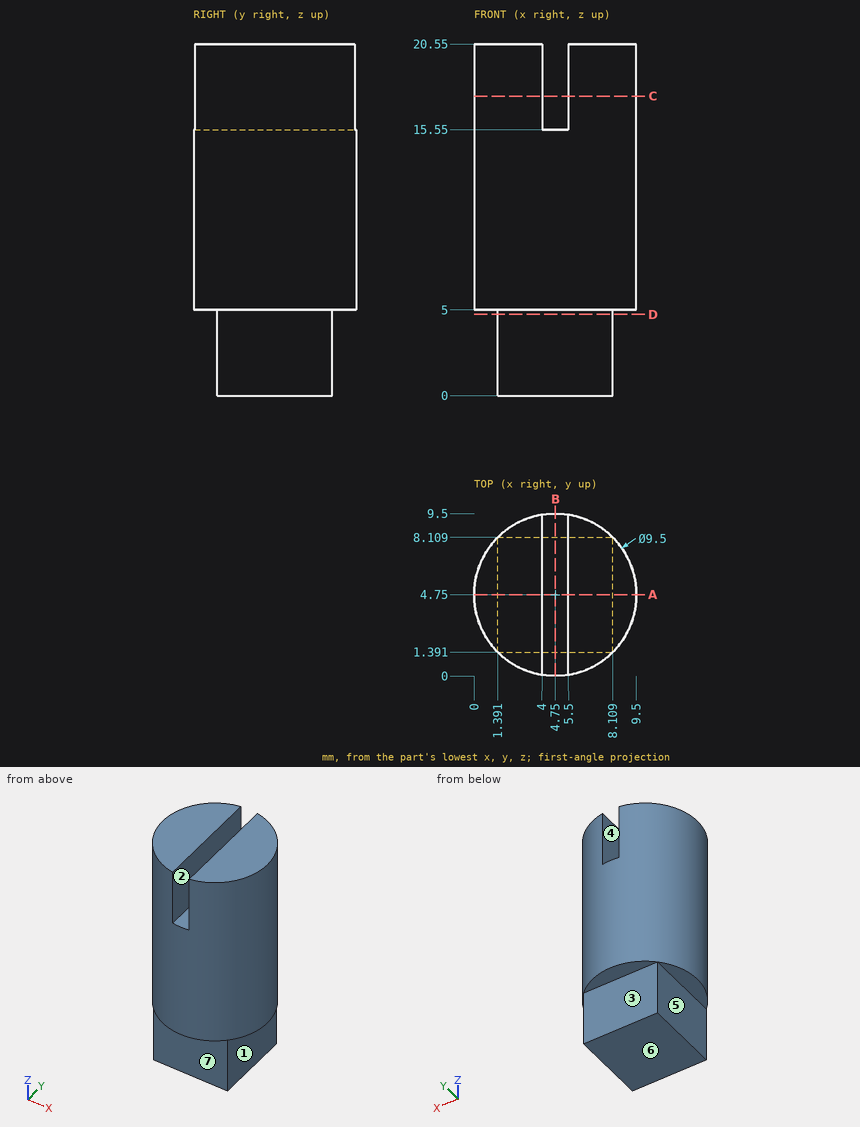
The figure shows three views and two pictorial views of one solid part (mm, origin at its lowest corner). Answer the questions. A direction names the side the tool comes from. Round coordinates to 2 decimals unless told otherwise and drop trailing zeros. Write each loop counter-clockwise with the first axis right and the second up, starting at its lowest first coordinate (ties: lowest second). Pieces come first, ordered by that corner, then holes. Notation, with made-up numbers: (22.5, 36.5) - (70.5, 36.5) arc R21 cw to (70.5, 53.5) - close; hole circle Ø1 at (54.25, 65). An arc over 180 degrees is marked (long way). Use one line per item in the form item = value. Start each with the question number.
Item 1: A cutting plane is placed at A-A (y = 4.75). Write down the section's boundary in (x, z), plus the area to 3 significant figures.
Item 2: Find the intervals of material crossed by line 1 (Z direction, x = 1.25, y = 2.25); line 2 (X direction, y = 8.25, z = 16.75); line 3 (Y direction, x = 1.5, z = 1.75), in increasing order. Write a range as [from, to].
Item 3: A cutting plane is placed at C-C (z = 17.5). Write down the section's boundary in (x, y), plus the area to 3 significant figures.
Item 4: A cutting plane is placed at B-B (x = 4.75). Write down the section's boundary in (y, z), plus the area to 3 significant figures.
Item 5: Determine the mould class of the marked faces 1, 2, 3 and 4 for opening direction X: +X half, -X half, draft (parallel to the pull), parting line (faces both ways), or undercut.
Item 6: Flat-ended cylindrical pins translate along their axes: pin 1 Ø1 at (y, z) = (3, 6.5) entering from +X; pin 2 Ø5 at (x, z) = (5, 4.5) entering from +Y; pin 3 Ø4 at (x, z) = (4, 2) entering from -Y; pin 4 Ø1.5 at (x, z) = (8.5, 9.5) entering from +Y. Find the tip coordinate at first contact, or state that the pin passes through.
Item 7: A tool of negligible diameter and unlimited length cuts with its end or side. For the marked faces 5, 6 and 7, from which of +Z, -Z, +X, -X, +Y, -Y can it reach the whole face along a straight path? Write none if from no direction.
Item 8: A cutting plane is placed at D-D (z = 4.75). Write down the section's boundary in (x, y).
The answers:
q1.outline = (0, 5) - (1.39, 5) - (1.39, 0) - (8.11, 0) - (8.11, 5) - (9.5, 5) - (9.5, 20.55) - (5.5, 20.55) - (5.5, 15.55) - (4, 15.55) - (4, 20.55) - (0, 20.55) - close
q1.area = 174 mm^2
q2.line_1 = [5, 20.55]
q2.line_2 = [1.54, 4], [5.5, 7.96]
q2.line_3 = [1.39, 8.11]
q3.outline = (4, 0.06) - (4, 9.44) arc R4.75 ccw to start; (5.5, 0.06) arc R4.75 ccw to (5.5, 9.44) - close
q3.area = 56.7 mm^2
q4.outline = (0, 5) - (1.39, 5) - (1.39, 0) - (8.11, 0) - (8.11, 5) - (9.5, 5) - (9.5, 15.55) - (0, 15.55) - close
q4.area = 134 mm^2
q5.face_1 = +X half
q5.face_2 = undercut
q5.face_3 = draft
q5.face_4 = undercut
q6.pin_1 = 9.33
q6.pin_2 = 9.5
q6.pin_3 = 1.39
q6.pin_4 = 8.43
q7.face_5 = -Z, -X, +Y, -Y
q7.face_6 = -Z, +X, -X, +Y, -Y
q7.face_7 = -Z, +X, -X, -Y
q8.outline = (1.39, 1.39) - (8.11, 1.39) - (8.11, 8.11) - (1.39, 8.11) - close
